Work out the finished part from the listing and answer in its coordinate system (mm). Face numbers are marked on the shaded views. A direction names the side the tool comes from. Round coordinates to 2 decimals unless told otherwise and drop trailing zeros. Order: outer loops, then holes, each group sorted by start corner. A loop starts at its lowest first (then second) coordinate and runs counter-clockwise, first axis right, second up. Notation, with made-up numbers: M 10.5,34.25 L 43.5,34.25 A8 cw 43.5,49.25 Z; hole C -24.5,-10 d11. An arc over 180 degrees is marked long. Return JSON: item names as keys, results as strings.
from build123d import *

# Parameters (mm, degrees)
SKETCH1_W           = 50
SKETCH1_H           = 18
BOSS_EXTRUDE1_DEPTH = 7
SKETCH2_W           = 50
SKETCH2_H           = 8
BOSS_EXTRUDE2_DEPTH = 33.5
SKETCH3_W           = 7
SKETCH3_H           = 8
BOSS_EXTRUDE3_DEPTH = 23
SKETCH4_W           = 7
SKETCH4_H           = 8
BOSS_EXTRUDE4_DEPTH = 14
SKETCH5_W           = 50
SKETCH5_H           = 10
CUT_EXTRUDE1_DEPTH  = 14
SKETCH6_R           = 2
CUT_EXTRUDE2_DEPTH  = 14
SKETCH7_W           = 50
SKETCH7_H           = 6
BOSS_EXTRUDE5_DEPTH = 67.91
CUT_EXTRUDE3_DEPTH  = 35
SKETCH9_R           = 2
CUT_EXTRUDE5_DEPTH  = 35
BOSS_EXTRUDE8_DEPTH = 50
SKETCH13_W          = 14
SKETCH13_H          = 8
CUT_EXTRUDE6_DEPTH  = 10


with BuildPart() as part:
    # Sketch1 → Boss-Extrude1 (new body)
    with BuildSketch(Plane.XY):
        with Locations((-12.394067797, 1.955508475)):
            Rectangle(SKETCH1_W, SKETCH1_H)
    extrude(amount=BOSS_EXTRUDE1_DEPTH)

    # Sketch2 → Boss-Extrude2 (add)
    with BuildSketch(Plane.XY.offset(7)):
        with Locations((-12.394067797, 6.955508475)):
            Rectangle(SKETCH2_W, SKETCH2_H)
    extrude(amount=BOSS_EXTRUDE2_DEPTH)

    # Sketch3 → Boss-Extrude3 (add)
    with BuildSketch(Plane(origin=(12.605932203, 0, 0), x_dir=(0, 0, -1), z_dir=(1, 0, 0))):
        with Locations((-3.5, 6.955508475)):
            Rectangle(SKETCH3_W, SKETCH3_H)
    extrude(amount=BOSS_EXTRUDE3_DEPTH)

    # Sketch4 → Boss-Extrude4 (add)
    with BuildSketch(Plane.ZY.offset(37.394067797)):
        with Locations((3.5, 6.955508475)):
            Rectangle(SKETCH4_W, SKETCH4_H)
    extrude(amount=BOSS_EXTRUDE4_DEPTH)

    # Sketch5 → Cut-Extrude1 (cut)
    with BuildSketch(Plane.XY.offset(7)):
        with Locations((-12.394067797, -2.044491525)):
            Rectangle(SKETCH5_W, SKETCH5_H)
    extrude(amount=-CUT_EXTRUDE1_DEPTH, mode=Mode.SUBTRACT)

    # Sketch6 → Cut-Extrude2 (cut)
    with BuildSketch(Plane.XY.offset(7)):
        with Locations((19.605932203, 6.955508475)):
            Circle(SKETCH6_R)
        with Locations((28.605932203, 6.955508475)):
            Circle(SKETCH6_R)
    extrude(amount=-CUT_EXTRUDE2_DEPTH, mode=Mode.SUBTRACT)

    # Sketch7 → Boss-Extrude5 (add)
    with BuildSketch(Plane.XZ.offset(-2.955508475)):
        with Locations((-12.394067797, 37.5)):
            Rectangle(SKETCH7_W, SKETCH7_H)
    extrude(amount=BOSS_EXTRUDE5_DEPTH)

    # Sketch8 → Cut-Extrude3 (cut)
    with BuildSketch(Plane.XY.offset(40.5)):
        with BuildLine():
            Line((-4.394067797, -44.33115583), (-4.394067797, -64.954491525))
            ThreePointArc((-4.394067797, -64.954491525), (-12.394067797, -72.954491525), (-20.394067797, -64.954491525))
            Line((-20.394067797, -64.954491525), (-20.394067797, -44.33115583))
            ThreePointArc((-20.394067797, -44.33115583), (-12.394067797, -36.33115583), (-4.394067797, -44.33115583))
        make_face()
    extrude(amount=-CUT_EXTRUDE3_DEPTH, mode=Mode.SUBTRACT)

    # Sketch9 → Cut-Extrude5 (cut)
    with BuildSketch(Plane(origin=(0, 0, 34.5), x_dir=(-1, 0, 0), z_dir=(0, 0, -1))):
        with Locations((27.901028765, -41.756933891)):
            Circle(SKETCH9_R)
        with Locations((4.616687569, -28.370715783)):
            Circle(SKETCH9_R)
    extrude(amount=-CUT_EXTRUDE5_DEPTH, mode=Mode.SUBTRACT)

    # Sketch12 → Boss-Extrude8 (add)
    with BuildSketch(Plane.ZY.offset(37.394067797)):
        Polygon((34.5, -1.873493289), (29.5872605, 2.955508475), (34.5, 2.955508475), align=None)
    extrude(amount=-BOSS_EXTRUDE8_DEPTH)

    # Sketch13 → Cut-Extrude6 (cut)
    with BuildSketch(Plane.XY.offset(7)):
        with Locations((-44.394067797, 6.955508475)):
            Rectangle(SKETCH13_W, SKETCH13_H)
    extrude(amount=-CUT_EXTRUDE6_DEPTH, mode=Mode.SUBTRACT)


solid = part.part
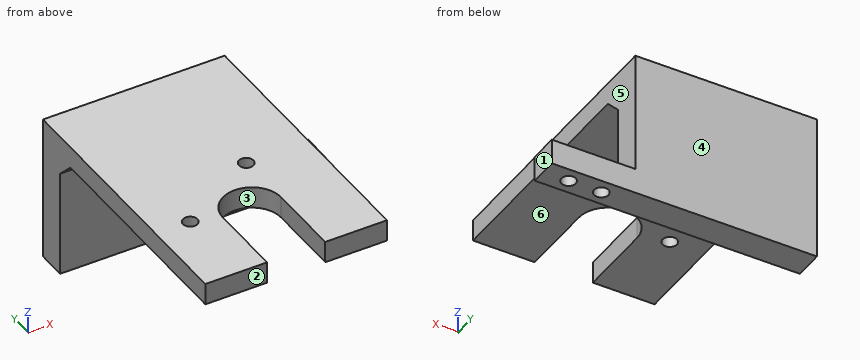
Item 1: Find section C-C (z = 38.5). Determine the outline of the cut face in (x, y).
Output:
{"outline": "M -37.39,-64.95 L -20.39,-64.95 L -20.39,-44.33 A8 cw -4.39,-44.33 L -4.39,-64.95 L 12.61,-64.95 L 12.61,10.96 L -37.39,10.96 Z; hole C -27.9,-41.76 d4; hole C -4.62,-28.37 d4"}
Item 2: Each of these flat-tipped pins is pushed along its axis until it touches: pin 1 (3 mm diameter, centred on x = -2.5, z = 32.5, fed in from -Y); pin 2 (15 mm diameter, centred on x = -8.5, y = -22, fed in from -Z); pin 3 (1 mm diameter, centred on x = -23.5, z = 28, fed in from -Y). Where does it stop, or does it pass through?
Output:
{"pin 1": "stops at y = -1.38", "pin 2": "stops at z = 34.5", "pin 3": "stops at y = 2.96"}
Item 3: Which of the six approach directions +Z, -Z, +X, -X, +Y, -Y give full straight-line access (tool end or side, diameter ignored) to the marked faces 4, 5 and 6?
Output:
{"face 4": "+Z, -Z, +X, -X, +Y", "face 5": "+Z, +X, +Y, -Y", "face 6": "-Z, +X, -X, -Y"}
Item 4: The mould has two halves that part along X. Classify the marked faces 1, 2 and 3: pulls with the +X half, pulls with the -X half, needs draft (parallel to the pull), parting line crosses it, or undercut.
Output:
{"face 1": "pulls with the +X half", "face 2": "needs draft", "face 3": "undercut"}
Item 5: Find section A-A (y = -46). Determine the outline of the cut face in (x, z).
Output:
{"outline": "M -37.39,34.5 L -20.39,34.5 L -20.39,40.5 L -37.39,40.5 Z; M -4.39,34.5 L 12.61,34.5 L 12.61,40.5 L -4.39,40.5 Z"}
Item 6: Find section B-B (x = 28.5). Determine the outline of the cut face in (y, z).
Output:
{"outline": "M 2.96,0 L 4.96,0 L 4.96,7 L 2.96,7 Z; M 8.95,0 L 10.96,0 L 10.96,7 L 8.95,7 Z"}
Item 7: Find section D-D (x = 5). Determine the outline of the cut face in (y, z).
Output:
{"outline": "M -64.95,34.5 L -1.87,34.5 L 2.96,29.59 L 2.96,0 L 10.96,0 L 10.96,40.5 L -64.95,40.5 Z"}
Item 8: Consider line 1 along X through (y, z) = (-61, 35); line 2 along Z through (x, y) = (1.5, -17); line 3 along Y through (x, z) = (-32, 5.5). Determine where each line is inside the solid, lowest interval first. Write a range as [from, to].
Output:
{"line 1": "x = [-37.39, -20.39], [-4.39, 12.61]", "line 2": "z = [34.5, 40.5]", "line 3": "y = [2.96, 10.96]"}
